Autodesk Inventor part; units mm, degrees
ref_plane "YZ Plane" through (0, 0, 0) normal (1, 0, 0) x (0, 1, 0)
ref_plane "XZ Plane" through (0, 0, 0) normal (0, 1, 0) x (-1, 0, 0)
ref_plane "XY Plane" through (0, 0, 0) normal (0, 0, 1) x (1, 0, 0)
sketch "Sketch1" plane through (0, 0, 0) normal (0, 1, 0) x (-1, 0, 0)
  line L0 (0, 0) -> (24.226, 0)
  line L1 (24.226, 0) -> (24.226, -140)
  line L2 (24.226, -140) -> (0, -140)
  line L3 (0, -140) -> (0, 0)
  dimension "d0" = 24.226
  dimension "d1" = 140
extrude "Extrusion1" add sketch "Sketch1" along normal blind 5
sketch "Sketch2" plane through (0, 5, 0) normal (0, 1, 0) x (1, 0, 0)
  point P0 (0, 0)
sketch "Sketch3" plane through (0, 0, 0) normal (0, -1, 0) x (1, 0, 0)
  circle A0 centre (-12.113, -2.5) radius 1.5
  point P0 (0, 0)
  dimension "d4" = 3
extrude "Extrusion2" add sketch "Sketch3" along normal blind 2
sketch "Sketch4" plane through (0, 0, 0) normal (0, -1, 0) x (1, 0, 0)
  point P0 (0, 0)
sketch "Sketch5" plane through (-12.113, -2, -2.5) normal (0, -1, 0) x (1, 0, 0)
  line L0 (-0.5, 1.5) -> (0.5, 1.5)
  line L1 (0.5, 1.5) -> (0.5, -1.5)
  line L2 (0.5, -1.5) -> (-0.5, -1.5)
  line L3 (-0.5, -1.5) -> (-0.5, 1.5)
  line L4 (-0.5, 1.5) -> (0.5, -1.5) construction
  line L5 (0.5, 1.5) -> (-0.5, -1.5) construction
  point P0 (12.113, 2.5)
  point P1 (0, 0)
  dimension "d7" = 1
extrude "Extrusion3" cut sketch "Sketch5" against normal blind 1.5
pattern_linear "Rectangular Pattern1" count 2 spacing 135 along (0, 0, -1) of "Extrusion2", "Extrusion3"
properties part number "part 2 upper part"
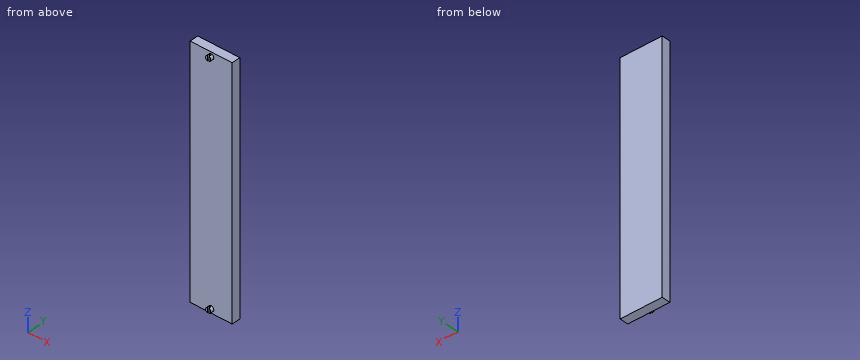
Check sheet for the modelled part. Datum: model origin and axes. Units: mm. Give positions to 0.01 mm unless a question says otherwise; leave off trailing zeros. Order: outer loops, then holes, each group sorted by start corner. A loop starts at its lowest first (then second) coordinate and runs counter-clockwise, first axis right, second up. Notation, with made-up numbers: (-33, -3) -> (-19, -3) arc R13 cw to (-19, 12) -> close; hole circle Ø11 at (-14.5, -33.75). An arc over 180 degrees is marked (long way). Return JSON: item names as keys, results as strings.
1. Cross-section at A-A, the plane z = -2.5. Record the cut outline in (x, y).
From the geometry:
{"outline": "(-24.23, 0) -> (-13.61, 0) -> (-13.61, -2) -> (-12.61, -2) -> (-12.61, -0.5) -> (-11.61, -0.5) -> (-11.61, -2) -> (-10.61, -2) -> (-10.61, 0) -> (0, 0) -> (0, 5) -> (-24.23, 5) -> close"}
2. Material ranges on probe 1 along Y at (x, z) = (-6, -131), recorded low to high. Write a range as [from, to].
From the geometry:
{"probe 1": "[0, 5]"}
3. Go/stop test with flat-tipped pins: P1, Ø0.8, axis at x = -12.5, z = -138, coming from the -Y side; P2, Ø0.8, axis at y = -1.5, z = -138, coming from the +X side; P3, Ø7.5, axis at x = -8.5, z = -40, coming from the -Y side; P4, Ø1.2, axis at y = -1.5, z = -2.5, coming from the -X side. Record where each tip stops, or that it passes through.
From the geometry:
{"P1": "y = -2", "P2": "x = -10.62", "P3": "y = 0", "P4": "x = -13.61"}
4. Cross-section at C-C, the plane z = -91.5. Record the cut outline in (x, y).
From the geometry:
{"outline": "(-24.23, 0) -> (0, 0) -> (0, 5) -> (-24.23, 5) -> close"}
5. Cross-section at B-B, the plane x = -2.5. Record the cut outline in (y, z).
From the geometry:
{"outline": "(0, -140) -> (5, -140) -> (5, 0) -> (0, 0) -> close"}
